```python
from build123d import *

# Parameters (mm, degrees)
BOSS_EXTRUDE1_DEPTH     = 15
SKETCH3_3_W             = 50
SKETCH3_3_H             = 20
BOSS_EXTRUDE2_DEPTH     = 25
SKETCH3_4_W             = 50
SKETCH3_4_H             = 25
BOSS_EXTRUDE3_DEPTH     = 65
SKETCH3_6_W             = 50
SKETCH3_6_H             = 10
BOSS_EXTRUDE4_DEPTH     = 25
CUT_EXTRUDE1_DEPTH      = 86.732140997
CUT_EXTRUDE1_DEPTH_BACK = 86.732140997
BOSS_EXTRUDE5_DEPTH     = 5


with BuildPart() as part:
    # Sketch3 → Boss-Extrude1 (new body)
    with BuildSketch(Plane.XY):
        with BuildLine():
            ThreePointArc((-25, 25), (0, 50), (25, 25))
            Line((25, 25), (25, 20))
            Line((25, 20), (-25, 20))
            Line((-25, 20), (-25, 25))
        make_face()
        with BuildLine():
            Line((15, 25), (-15, 25))
            ThreePointArc((-15, 25), (0, 40), (15, 25))
        make_face(mode=Mode.SUBTRACT)
    extrude(amount=BOSS_EXTRUDE1_DEPTH)

    # Sketch3_3 → Boss-Extrude2 (add)
    with BuildSketch(Plane.XY):
        with Locations((0, 10)):
            Rectangle(SKETCH3_3_W, SKETCH3_3_H)
    extrude(amount=BOSS_EXTRUDE2_DEPTH)

    # Sketch3_4 → Boss-Extrude3 (add)
    with BuildSketch(Plane.XY):
        with Locations((0, -12.5)):
            Rectangle(SKETCH3_4_W, SKETCH3_4_H)
    extrude(amount=BOSS_EXTRUDE3_DEPTH)

    # Sketch3_6 → Boss-Extrude4 (add)
    with BuildSketch(Plane.XY):
        with Locations((0, -30)):
            Rectangle(SKETCH3_6_W, SKETCH3_6_H)
    extrude(amount=BOSS_EXTRUDE4_DEPTH)

    # Sketch5 → Cut-Extrude1 (cut, two sides: drawn at the far end of the back side and taken through both)
    with BuildSketch(Plane(origin=(0, 0, 0), x_dir=(1, 0, 0), z_dir=(0, 1, 0)).offset(-CUT_EXTRUDE1_DEPTH_BACK)):
        with BuildLine():
            Line((-15, -65), (15, -65))
            ThreePointArc((15, -65), (0, -50), (-15, -65))
        make_face()
    extrude(amount=CUT_EXTRUDE1_DEPTH + CUT_EXTRUDE1_DEPTH_BACK, mode=Mode.SUBTRACT)

    # Sketch6 → Boss-Extrude5 (add, symmetric)
    with BuildSketch(Plane(origin=(0, 0, 0), x_dir=(0, 0, -1), z_dir=(1, 0, 0))):
        Polygon((-25, 20), (-45, 0), (-25, 0), align=None)
    extrude(amount=BOSS_EXTRUDE5_DEPTH, both=True)


solid = part.part
```
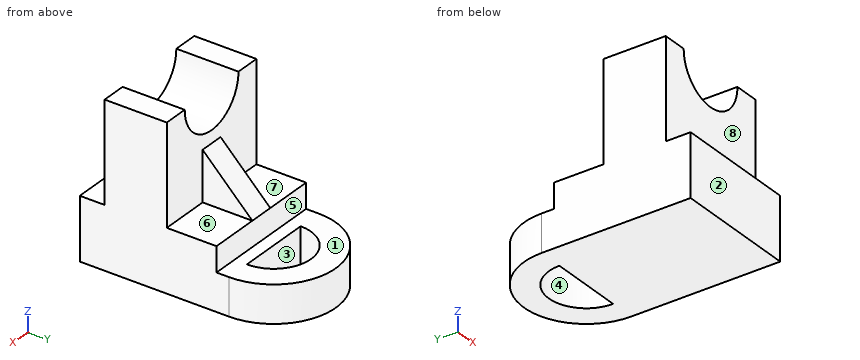
Input: part model. Units: mm. Frame: model coordinates. Face numbers are marked on the shaded views. A direction names the side the tool comes from. Coordinates: 2 decimals unless noted, no trailing zeros. Loops run counter-clockwise (first coordinate to the right, second up) from the corner with the lowest first, then second, coordinate; pieces in that order, holes last. Notation, with made-up numbers: M 80.5,43.5 L 119.5,43.5 A26 ccw 119.5,81.5 Z; hole C 40,48.25 d7. An arc over 180 degrees is marked long. Use a Markdown table: item, result. Add a question column.
1) Set-up query: the marked faces 4, 5, 6, 7 and 8. Return all of +Z, -Z, +X, -X, +Y, -Y with unobstructed straight access to the full face (end or side cutting, diameter ignored); none if empty.
2) Line query: L1, parallel to Z at x = -14, y = 23.5; L2, parallel to Y at x = -7, z = 49.5; L3, parallel to Z at x = -10.5, y = 1.5. Output: solid intervals per line, ascending. Write a range as from..to.
3) Pin query (flat end, axial travel): P1, Ø8, axis at x = 6, z = 35, coming from the -Y side; P2, Ø22, axis at y = 13.5, z = 37, coming from the -X side; P3, Ø24, axis at x = 8.5, y = 31, coming from the +Z side. Return the tip coordinate at first contact, or that it passes through.
4) Section C-C, the plane y = 37. Return the cut outline in (x, z), plus the area to 3 significant figures.
5) Draft query along Y for the marked faces 1, 2 and 3. Return one class per face: +Y half, -Y half, draft (parallel to the pull), parting line (faces both ways), or undercut.
6) Section D-D, the plane z = 54.5. Return the cut outline in (x, y), plus the area to 3 significant figures.
7) Section B-B, the plane z = 34. Return the cut outline in (x, y).
8) Section A-A, the plane x = 0. Return the cut outline in (y, z).
Answer below:
| question | item | result |
|---|---|---|
| 1 | face 4 | +Z, -Z |
| 1 | face 5 | +Z, +X, -X, +Y |
| 1 | face 6 | +Z, +X, +Y |
| 1 | face 7 | +Z, -X, +Y |
| 1 | face 8 | +Z, +X, -X, -Y |
| 2 | L1 | 0..15 |
| 2 | L2 | -25..0 |
| 2 | L3 | 0..25 |
| 3 | P1 | y = -25 |
| 3 | P2 | x = -5 |
| 3 | P3 | z = 25.48 |
| 4 | outline | M -21.93,0 L -9,0 L -9,15 L -21.93,15 Z; M 9,0 L 21.93,0 L 21.93,15 L 9,15 Z |
| 4 | area | 388 mm2 |
| 5 | face 1 | draft |
| 5 | face 2 | -Y half |
| 5 | face 3 | undercut |
| 6 | outline | M -25,-25 L -10.71,-25 L -10.71,0 L -25,0 Z; M 10.71,-25 L 25,-25 L 25,0 L 10.71,0 Z |
| 6 | area | 714 mm2 |
| 7 | outline | M -25,-25 L 25,-25 L 25,0 L 5,0 L 5,11 L -5,11 L -5,0 L -25,0 Z |
| 8 | outline | M -35,0 L 25,0 L 25,15 L 20,15 L 20,25 L 0,45 L 0,50 L -25,50 L -25,25 L -35,25 Z; M 40,0 L 50,0 L 50,15 L 40,15 Z |
